Here's how the part is built. I have some questions about the finished solid (model axes, mm). A direction names the side the tool comes from. Coordinates: 2 decimals unless noted, no trailing zeros. Loops run counter-clockwise (first coordinate to the right, second up) from the corner with the lowest first, then second, coordinate; pieces in that order, holes last. Notation, with made-up numbers: (-26, 51) - (-9, 51) arc R19 cw to (-9, 80) - close; hole circle Ø6 at (62, 41.5). An arc over 180 degrees is marked (long way). Use a Markdown table: item, result.
```python
from build123d import *

# Parameters (mm, degrees)
SKETCH2_W           = 1
SKETCH2_H           = 1
BOSS_EXTRUDE1_DEPTH = 5


with BuildPart() as part:
    # Sketch1 → Revolve1 (revolve)
    with BuildSketch(Plane(origin=(0, 0, 0), x_dir=(0, 0, -1), z_dir=(1, 0, 0))):
        with BuildLine():
            Line((0, 0), (0, 9.69))
            Line((0, 9.69), (-0.01, 9.69))
            ThreePointArc((-0.01, 9.69), (-1.770695885, 8.960695885), (-2.5, 7.2))
            Line((-2.5, 7.2), (-2.5, 1))
            Line((-2.5, 1), (-2.95, 1))
            Line((-2.95, 1), (-2.95, 0))
            Line((-2.95, 0), (0, 0))
        make_face()
    revolve(axis=Axis((0, 0, 0), (0, 1, 0)))

    # Sketch2 → Boss-Extrude1 (add)
    with BuildSketch(Plane.XZ):
        with Locations((-1.25, 0)):
            Rectangle(SKETCH2_W, SKETCH2_H)
        with Locations((1.25, 0)):
            Rectangle(SKETCH2_W, SKETCH2_H)
    extrude(amount=BOSS_EXTRUDE1_DEPTH)


solid = part.part
```
Q1. I want a section at A-A, the plane y = -3. Write out the boundary of the cut face in (x, z), then the cut area to 3 significant figures.
Check values:
| item | result |
|---|---|
| outline | (-1.75, -0.5) - (-0.75, -0.5) - (-0.75, 0.5) - (-1.75, 0.5) - close; (0.75, -0.5) - (1.75, -0.5) - (1.75, 0.5) - (0.75, 0.5) - close |
| area | 2.00 mm^2 |
Q2. If we mould it in two halves opening along X, with no side actions, what happens to faces 5 (the face through (0.13, 0.493, -2.947)), 6 (the face through (-1, -2, 0.5)), 7 (the face through (0.75, -2, 0)), 8 (the face through (1.75, -2, 0))? For each: pulls with the +X half, pulls with the -X half, needs draft (parallel to the pull), parting line crosses it, or undercut.
Check values:
| item | result |
|---|---|
| face 5 | parting line crosses it |
| face 6 | needs draft |
| face 7 | undercut |
| face 8 | pulls with the +X half |
Q3. Please list where these lines run through material, in increasing order: L1, parallel to Z at x = 0.05, y = 5.25; L2, parallel to Y at x = -0.7, z = -2.55; L3, parallel to Y at x = -0.7, z = -2.2. Write a range as from..to.
Check values:
| item | result |
|---|---|
| L1 | -2.5..2.5 |
| L2 | 0..1 |
| L3 | 0..8.16 |
Q4. Which directions (+Z, -Z, +X, -X, +Y, -Y) give clear straight access to the entire face, cutting with the end or side of a thin tool? Please do faces 1 (the face through (-1.75, -2, 0)), 2 (the face through (-1, -2, -0.5)), 3 (the face through (-0.75, -2, 0)), 4 (the face through (-2.44, 4.06, -0.54)).
Check values:
| item | result |
|---|---|
| face 1 | +Z, -Z, -X, -Y |
| face 2 | -Z, +X, -X, -Y |
| face 3 | +Z, -Z, -Y |
| face 4 | +Y |
Q5. I want a section at B-B, the plane y = 2. Write out the boundary of the cut face in (x, z), then the cut area to 3 significant figures.
Check values:
| item | result |
|---|---|
| outline | circle Ø5 at (0, 0) |
| area | 19.6 mm^2 |
Q6. Will these pins go through, and if not, where does the flat tip stop? P1, Ø1.5, axis at x = -2, y = 0.5, coming from the +Z side; P2, Ø0.5, axis at x = 1.5, y = -2.5, coming from the +Z side; P3, Ø1, axis at x = 2, y = 7.5, coming from the -Z side.
Check values:
| item | result |
|---|---|
| P1 | z = 2.67 |
| P2 | z = 0.5 |
| P3 | z = -1.98 |
